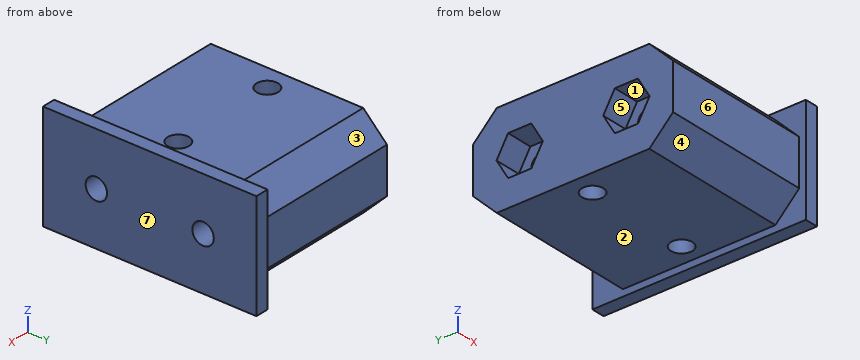
Autodesk Inventor part; units mm, degrees
ref_plane "YZ Plane" through (0, 0, 0) normal (1, 0, 0) x (0, 1, 0)
ref_plane "XZ Plane" through (0, 0, 0) normal (0, 1, 0) x (-1, 0, 0)
ref_plane "XY Plane" through (0, 0, 0) normal (0, 0, 1) x (1, 0, 0)
sketch "Sketch1" plane through (0, 0, 0) normal (1, 0, 0) x (0, 1, 0)
  line L0 (-23.8125, -11.1125) -> (23.8125, -11.1125)
  line L1 (23.8125, -11.1125) -> (23.8125, 11.1125)
  line L2 (23.8125, 11.1125) -> (-23.8125, 11.1125)
  line L3 (-23.8125, 11.1125) -> (-23.8125, -11.1125)
  line L4 (-23.8125, -11.1125) -> (23.8125, 11.1125) construction
  line L5 (23.8125, -11.1125) -> (-23.8125, 11.1125) construction
  line L6 (23.8125, 5.4556) -> (18.1556, 11.1125)
  line L7 (-18.1556, 11.1125) -> (-23.8125, 5.4556)
  line L8 (-18.1556, -11.1125) -> (-23.8125, -5.4556)
  line L9 (18.1556, -11.1125) -> (23.8125, -5.4556)
  point P0 (0, 0)
  dimension "d0" = 135
  dimension "d1" = 135
  dimension "d2" = 4
  dimension "d3" = 47.625
  dimension "d4" = 22.225
extrude "Extrusion1" add sketch "Sketch1" along normal blind 36 contours L8 L3 L7 L2 L6 L1 L9 L0
sketch "Sketch2" plane through (36, 0, 0) normal (1, 0, 0) x (0, 0, -1)
  line L0 (0, 12.7) -> (0, -12.7)
  point P0 (0, 0)
  point P1 (0, 0)
  dimension "d7" = 25.4
hole "Hole1" at (36, 12.7, 0) at (36, -12.7, 0) direction (-1, 0, 0) diameter 5.105 end through all
sketch "Sketch3" plane through (0, 0, 0) normal (-1, 0, 0) x (0, 0, 1)
  circle A0 centre (0, 12.7) radius 2.5525
  line L0 (-4.7752, 15.457) -> (0, 18.2139)
  line L1 (0, 18.2139) -> (4.7752, 15.457)
  line L2 (4.7752, 15.457) -> (4.7752, 9.943)
  line L3 (4.7752, 9.943) -> (0, 7.1861)
  line L4 (0, 7.1861) -> (-4.7752, 9.943)
  line L5 (-4.7752, 9.943) -> (-4.7752, 15.457)
  circle A1 centre (0, -12.7) radius 2.5525
  line L6 (-4.7752, -9.943) -> (0, -7.1861)
  line L7 (0, -7.1861) -> (4.7752, -9.943)
  line L8 (4.7752, -9.943) -> (4.7752, -15.457)
  line L9 (4.7752, -15.457) -> (0, -18.2139)
  line L10 (0, -18.2139) -> (-4.7752, -15.457)
  line L11 (-4.7752, -15.457) -> (-4.7752, -9.943)
  point P0 (0, 0)
  dimension "d15" = 9.5504
  dimension "d16" = 9.5504
extrude "Extrusion2" cut sketch "Sketch3" against normal blind 6.35 contours A0 | L0 L1 L2 L3 L4 L5 | A1 | L6 L7 L8 L9 L10 L11
sketch "Sketch4" plane through (36, 0, 0) normal (1, 0, 0) x (0, 0, -1)
  line L0 (12.7, -25.4) -> (-12.7, -25.4)
  line L1 (-12.7, -25.4) -> (-12.7, 25.4)
  line L2 (-12.7, 25.4) -> (12.7, 25.4)
  line L3 (12.7, 25.4) -> (12.7, -25.4)
  line L4 (12.7, -25.4) -> (-12.7, 25.4) construction
  line L5 (-12.7, -25.4) -> (12.7, 25.4) construction
  circle A0 centre (0, 12.7) radius 2.5525
  circle A1 centre (0, -12.7) radius 2.5525
  point P0 (0, 0)
  dimension "d19" = 25.4
  dimension "d20" = 50.8
extrude "Extrusion3" add sketch "Sketch4" along normal blind 3.175
sketch "Sketch5" plane through (0, -18.1556, 11.1125) normal (0, 0, 1) x (1, 0, 0)
  line L0 (36, 43.5556) -> (36, -7.2444)
  line L1 (0, 36.3113) -> (0, 0)
  point P0 (0, 18.1556)
  point P1 (31, 18.1556)
  point P2 (5.6, 18.1556)
  point P3 (0, 18.1556)
  dimension "d23" = 25.4
  dimension "d24" = 5
hole "Hole2" at (31, 0, 11.1125) at (5.6, 0, 11.1125) direction (0, 0, -1) diameter 5.105 end through all
equation "\"d1\" = d0"
equation "\"d16\" = d15"
properties part number "TUBE_PLUGS" material "3D Print Material - chopped carbon Nylon12 (preferred)"
Could you check a few things on this model? Use its own coordinates, in mm. Face numbers are marked on the shaded views. A direction names the side the tool comes from. Coordinates: 2 decimals unless noted, no trailing zeros. Loops run counter-clockwise (first coordinate to the right, second up) from the corner with the lowest first, then second, coordinate; pieces in that order, holes last. Notation, with made-up numbers: (28, 61) -> (63, 61) arc R15 cw to (63, 80) -> close; hole circle Ø11 at (52, 39.5). An arc over 180 degrees is marked (long way). Answer in a Markdown table with one row per item.
(1) Thinking about a two-plate mould opening in Y: for the marked faces 5, 6 and 7, which applies, released by +Y, released by -Y, zero draft, split by the parting line, or undercut?
Results found:
| item | result |
|---|---|
| face 5 | undercut |
| face 6 | released by -Y |
| face 7 | zero draft |
(2) For the marked faces 1, 2, 3 and 4, which set-ups out of +Z, -Z, +X, -X, +Y, -Y let a thin tool reach every point of the face, with its end or its side?
Results found:
| item | result |
|---|---|
| face 1 | -X |
| face 2 | -Z, -X, +Y, -Y |
| face 3 | +Z, -X, +Y |
| face 4 | -Z, -X, -Y |
(3) Will these pins go through, and if not, where does the flat tip stop? pin 1 Ø4 at (x, z) = (16.5, 5.5) entering from +Y; pin 2 Ø3 at (x, y) = (1.5, 12) entering from +Z; pin 3 Ø4 at (x, y) = (31, 0) entering from -Z; pin 4 Ø10 at (x, y) = (24.5, 5.5) entering from -Z.
Results found:
| item | result |
|---|---|
| pin 1 | stops at y = 23.81 |
| pin 2 | stops at z = 11.11 |
| pin 3 | passes through |
| pin 4 | stops at z = -11.11 |
(4) Imagine slicing it at B-B (y = 0). List the corners of the cut face in (x, z) for me (1 decimal).
Results found:
| item | result |
|---|---|
| outline | (0, -11.1) -> (3, -11.1) -> (3, 11.1) -> (0, 11.1) -> close; (8.2, -11.1) -> (28.4, -11.1) -> (28.4, 11.1) -> (8.2, 11.1) -> close; (33.6, -11.1) -> (36, -11.1) -> (36, -12.7) -> (39.2, -12.7) -> (39.2, 12.7) -> (36, 12.7) -> (36, 11.1) -> (33.6, 11.1) -> close |
(5) If I drill on probe 1 along X at (y, z) = (0, -7.5) (1 decimal); probe 2 along Y at (x, z) = (31, 0); probe 3 along Y at (x, z) = (25.5, 0), over which ranges is the centre line in solid material (lowest first)?
Results found:
| item | result |
|---|---|
| probe 1 | x = 0 to 3, 8.2 to 28.4, 33.6 to 39.2 |
| probe 2 | y = -23.81 to -15.25, -10.15 to -2.55, 2.55 to 10.15, 15.25 to 23.81 |
| probe 3 | y = -23.81 to -15.25, -10.15 to 10.15, 15.25 to 23.81 |
(6) Imagine slicing it at C-C (x = 25). List the corners of the cut face in (y, z) for me (1 decimal).
Results found:
| item | result |
|---|---|
| outline | (-23.8, -5.5) -> (-18.2, -11.1) -> (18.2, -11.1) -> (23.8, -5.5) -> (23.8, 5.5) -> (18.2, 11.1) -> (-18.2, 11.1) -> (-23.8, 5.5) -> close; hole circle Ø5.1 at (-12.7, 0); hole circle Ø5.1 at (12.7, 0) |
(7) Imagine slicing it at A-A (x = 5.6). List the corners of the cut face in (y, z) for me.
Results found:
| item | result |
|---|---|
| outline | (-23.81, -5.46) -> (-18.16, -11.11) -> (-2.55, -11.11) -> (-2.55, 11.11) -> (-18.16, 11.11) -> (-23.81, 5.46) -> close; (2.55, -11.11) -> (18.16, -11.11) -> (23.81, -5.46) -> (23.81, 5.46) -> (18.16, 11.11) -> (2.55, 11.11) -> close; hole (-18.21, 0) -> (-15.46, -4.78) -> (-9.94, -4.78) -> (-7.19, 0) -> (-9.94, 4.78) -> (-15.46, 4.78) -> close; hole (7.19, 0) -> (9.94, -4.78) -> (15.46, -4.78) -> (18.21, 0) -> (15.46, 4.78) -> (9.94, 4.78) -> close |
